```python
from build123d import *

# Parameters (mm, degrees)
SKETCH_1_W          = 116
SKETCH_1_H          = 50
EXTRUDE_1_DEPTH     = 2
CHAMFER_1_SIZE      = 2
SKETCH_2_W          = 2
SKETCH_2_H          = 25.2
CUT_EXTRUDE_1_DEPTH = 127.332893579


with BuildPart() as part:
    # 草图1 → 凸台-拉伸1 (new body)
    with BuildSketch(Plane.XY):
        with Locations((58, -25)):
            Rectangle(SKETCH_1_W, SKETCH_1_H)
    extrude(amount=EXTRUDE_1_DEPTH)

    # 倒角1
    chamfer_1_edges = [part.edges().sort_by_distance(p)[0] for p in [
        (116, -50, 1),
        (0, -50, 1),
    ]]
    chamfer(chamfer_1_edges, length=CHAMFER_1_SIZE)

    # 草图2 → 切除-拉伸1 (cut, through all)
    with BuildSketch(Plane(origin=(0, 0, 0), x_dir=(-1, 0, 0), z_dir=(0, 0, -1))):
        with Locations((-58, -37.4)):
            Rectangle(SKETCH_2_W, SKETCH_2_H)
    extrude(amount=-CUT_EXTRUDE_1_DEPTH, mode=Mode.SUBTRACT)


solid = part.part
```
Geometry: final body of the model. Coordinates: model frame, mm. A direction names the side the tool comes from. Round coordinates to 2 decimals unless told otherwise and drop trailing zeros. Write each loop counter-clockwise with the first axis right and the second up, starting at its lowest first coordinate (ties: lowest second). Pieces come first, ordered by that corner, then holes.
Item 1: Material intervals for L1, parallel to X at y = -46, z = 1.45, sorted ascending.
Item 2: Mould query, pull axis X, two halves, no side actions, for faces 1 (the face through (58, -24.8, 1)), 2 (the face through (57.2, -24.6, 2)), 3 (the face through (115, -49, 1)). Classes: +X half, -X half, draft (parallel to the pull), parting line (faces both ways), or undercut.
Item 3: Section query A-A (y = -32). Return loops of the section in (x, z).
Item 4: Set-up query: faces 4 (the face through (116, -24, 1)), 5 (the face through (57, -38, 1)). Return all of +Z, -Z, +X, -X, +Y, -Y with unobstructed straight access to the full face (end or side cutting, diameter ignored); none if empty.
Item 5: Pin query (flat end, axial travel): P1, Ø0.6, axis at x = 58, z = 1.5, coming from the -Y side. Return the tip coordinate at first contact, or that it passes through.
Completed:
1. L1: x = 0 to 57, 59 to 116
2. face 1: undercut
2. face 2: draft
2. face 3: +X half
3. outline: (0, 0) - (57, 0) - (57, 2) - (0, 2) - close; (59, 0) - (116, 0) - (116, 2) - (59, 2) - close
4. face 4: +Z, -Z, +X, +Y, -Y
4. face 5: +Z, -Z, -Y
5. P1: stops at y = -24.8
